from build123d import *

# Parameters (mm, degrees)
SKETCH_1_R          = 1.5
SKETCH_1_R_2        = 1.95
SKETCH_1_R_3        = 10
EXTRUDE_1_DEPTH     = 3
SKETCH_2_R          = 1.5
CUT_EXTRUDE_1_DEPTH = 131.395552071


with BuildPart() as part:
    # 草图1 → 凸台-拉伸1 (new body)
    with BuildSketch(Plane(origin=(0, 0, 0), x_dir=(1, 0, 0), z_dir=(0, 1, 0))):
        with BuildLine():
            Line((-108, -65), (60, -65))
            ThreePointArc((60, -65), (63.535533906, -63.535533906), (65, -60))
            Line((65, -60), (65, 60))
            ThreePointArc((65, 60), (63.535533906, 63.535533906), (60, 65))
            Line((60, 65), (-108, 65))
            ThreePointArc((-108, 65), (-111.535533906, 63.535533906), (-113, 60))
            Line((-113, 60), (-113, -60))
            ThreePointArc((-113, -60), (-111.535533906, -63.535533906), (-108, -65))
        make_face()
        with Locations(Location((0, 45, 0), (0, 0, 270))):
            Circle(SKETCH_1_R, mode=Mode.SUBTRACT)
        with Locations(Location((-38.97114317, -22.5, 0), (0, 0, 270))):
            Circle(SKETCH_1_R, mode=Mode.SUBTRACT)
        with Locations(Location((38.97114317, -22.5, 0), (0, 0, 270))):
            Circle(SKETCH_1_R, mode=Mode.SUBTRACT)
        with Locations(Location((-45, 0, 0), (0, 0, 270))):
            Circle(SKETCH_1_R_2, mode=Mode.SUBTRACT)
        with Locations(Location((45, 0, 0), (0, 0, 270))):
            Circle(SKETCH_1_R_2, mode=Mode.SUBTRACT)
        with Locations(Location((-95, -27.5, 0), (0, 0, 270))):
            Circle(SKETCH_1_R, mode=Mode.SUBTRACT)
        with Locations(Location((-60.1, -27.5, 0), (0, 0, 90))):
            Circle(SKETCH_1_R, mode=Mode.SUBTRACT)
        with Locations(Location((-77.55, 23, 0), (0, 0, 270))):
            Circle(SKETCH_1_R, mode=Mode.SUBTRACT)
        with Locations(Location((-108, 60, 0), (0, 0, 270))):
            Circle(SKETCH_1_R, mode=Mode.SUBTRACT)
        with Locations(Location((60, 60, 0), (0, 0, 270))):
            Circle(SKETCH_1_R, mode=Mode.SUBTRACT)
        with Locations(Location((60, -60, 0), (0, 0, 270))):
            Circle(SKETCH_1_R, mode=Mode.SUBTRACT)
        with Locations(Location((-108, -60, 0), (0, 0, 270))):
            Circle(SKETCH_1_R, mode=Mode.SUBTRACT)
        with Locations(Location((0, -32, 0), (0, 0, 270))):
            Circle(SKETCH_1_R_3, mode=Mode.SUBTRACT)
    extrude(amount=EXTRUDE_1_DEPTH)

    # 草图2 → 切除-拉伸1 (cut, through all)
    with BuildSketch(Plane(origin=(0, 3, 0), x_dir=(1, 0, 0), z_dir=(0, 1, 0))):
        with Locations(Location((-87.55, 62, 0), (0, 0, 270))):
            Circle(SKETCH_2_R)
        with Locations(Location((-67.55, 62, 0), (0, 0, 270))):
            Circle(SKETCH_2_R)
        with Locations(Location((-77.55, 38.3, 0), (0, 0, 270))):
            Circle(SKETCH_2_R)
    extrude(amount=-CUT_EXTRUDE_1_DEPTH, mode=Mode.SUBTRACT)


solid = part.part
Verification items for the finished model (mm, model axes). Give positions to 0.01 mm unless a question says otherwise; leave off trailing zeros. Write each loop counter-clockwise with the first axis right and the second up, starting at its lowest first coordinate (ties: lowest second). Pieces come first, ordered by that corner, then holes.
(1) Cross-section at A-A (z = 32). Enter the section's corners in (x, y), plus the area to 3 significant figures.
(2) Mould release check, pull along Z, two halves, no side actions. Record for faces 1 (the face through (64, 1, -63)), 2 (the face through (-112, 1, 63)), 3 (the face through (-46.904, 1.479, -0.423)), 4 (the face through (3, 1.48, 41.54)): +Z half, -Z half, draft (parallel to the pull), parting line (faces both ways), or undercut.
(3) Cross-section at C-C (y = 0.95). State how many separate pieces and enclosed holes the cut face has, plus the area to 3 significant figures.
(4) Material ranges on line 1 (Z direction, x = -108, y = 2.15); line 2 (X direction, y = 0.95, z = 0); line 3 (X direction, y = 1.2, z = -60), recorded low to high.
(5) Cross-section at B-B (x = 45). Enter the section's corners in (y, z).
Worked out:
1. outline: (-113, 0) - (-10, 0) - (-10, 3) - (-113, 3) - close; (10, 0) - (65, 0) - (65, 3) - (10, 3) - close
1. area: 474 mm2
2. face 1: -Z half
2. face 2: +Z half
2. face 3: undercut
2. face 4: undercut
3. separate pieces: 1
3. enclosed holes: 16
3. area: 22,700 mm2
4. line 1: z = -65 to -61.5, -58.5 to 58.5, 61.5 to 65
4. line 2: x = -113 to -46.95, -43.05 to 43.05, 46.95 to 65
4. line 3: x = -113 to -109.5, -106.5 to 58.5, 61.5 to 65
5. outline: (0, -65) - (3, -65) - (3, -1.95) - (0, -1.95) - close; (0, 1.95) - (3, 1.95) - (3, 65) - (0, 65) - close
